Geometry check sheet. Reference: the model listing, model coordinates, mm. A direction names the side the tool comes from. Give positions to 0.01 mm unless a question says otherwise; leave off trailing zeros. Write each loop counter-clockwise with the first axis right and the second up, starting at its lowest first coordinate (ties: lowest second). Pieces come first, ordered by that corner, then holes. Notation, with made-up numbers: (52, 81.5) - (105, 81.5) arc R6 cw to (105, 87.5) - close; hole circle Ø2 at (-37.5, 50). An arc over 180 degrees is marked (long way). Use a Markdown table: item, result.
```python
from build123d import *

# Parameters (mm, degrees)
BOX_W             = 43
BOX_H             = 27
BOX_DEPTH         = 10
CYLINDER001_R     = 15.5
CYLINDER001_DEPTH = 9
CYLINDER002_R     = 17.5
CYLINDER002_DEPTH = 2
CYLINDER_R        = 3.5
CYLINDER_DEPTH    = 10
CYLINDER003_R     = 5.5
CYLINDER003_DEPTH = 2
CYLINDER004_R     = 5
CYLINDER004_DEPTH = 10
BOX001_W          = 35
BOX001_H          = 2
BOX001_DEPTH      = 2
CHAMFER_SIZE      = 1
CHAMFER001_SIZE   = 0.9
CHAMFER002_SIZE   = 1
CHAMFER003_SIZE   = 0.9
CHAMFER004_SIZE   = 0.5


with BuildPart() as cube:
    # Box → Box (new body)
    with BuildSketch(Plane(origin=(-22, 0, -1), x_dir=(1, 0, 0), z_dir=(0, 0, 1))):
        with Locations((21.5, 13.5)):
            Rectangle(BOX_W, BOX_H)
    extrude(amount=BOX_DEPTH)


with BuildPart() as cylinder001:
    # Cylinder001 → Cylinder001 (new body)
    with BuildSketch(Plane.XY.offset(-1)):
        Circle(CYLINDER001_R)
    extrude(amount=CYLINDER001_DEPTH)


with BuildPart() as cut001:
    # Cylinder002 → Cylinder002 (new body)
    with BuildSketch(Plane.XY):
        Circle(CYLINDER002_R)
    extrude(amount=CYLINDER002_DEPTH)

    # Cut: cut Cylinder001
    add(cylinder001.part, mode=Mode.SUBTRACT)

    # Cut001: cut Cube
    add(cube.part, mode=Mode.SUBTRACT)


with BuildPart() as cylinder:
    # Cylinder → Cylinder (new body)
    with BuildSketch(Plane.XY.offset(-3)):
        Circle(CYLINDER_R)
    extrude(amount=CYLINDER_DEPTH)


with BuildPart() as cut002:
    # Cylinder003 → Cylinder003 (new body)
    with BuildSketch(Plane.XY):
        Circle(CYLINDER003_R)
    extrude(amount=CYLINDER003_DEPTH)

    # Cut002: cut Cylinder
    add(cylinder.part, mode=Mode.SUBTRACT)


with BuildPart() as cylinder004:
    # Cylinder004 → Cylinder004 (new body)
    with BuildSketch(Plane.XY.offset(-3)):
        Circle(CYLINDER004_R)
    extrude(amount=CYLINDER004_DEPTH)


with BuildPart() as prop_guard:
    # Box001 → Box001 (new body)
    with BuildSketch(Plane(origin=(-17.5, -2, 0), x_dir=(1, 0, 0), z_dir=(0, 0, 1))):
        with Locations((17.5, 1)):
            Rectangle(BOX001_W, BOX001_H)
    extrude(amount=BOX001_DEPTH)

    # Cut003: cut Cylinder004
    add(cylinder004.part, mode=Mode.SUBTRACT)

    # Chamfer
    chamfer_edges = [prop_guard.edges().sort_by_distance(p)[0] for p in [
        (11.25, 0, 2),
    ]]
    chamfer(chamfer_edges, length=CHAMFER_SIZE)

    # Chamfer001
    chamfer001_edges = [prop_guard.edges().sort_by_distance(p)[0] for p in [
        (11.041288, -2, 2),
    ]]
    chamfer(chamfer001_edges, length=CHAMFER001_SIZE)

    # Chamfer002
    chamfer002_edges = [prop_guard.edges().sort_by_distance(p)[0] for p in [
        (-11.25, 0, 2),
    ]]
    chamfer(chamfer002_edges, length=CHAMFER002_SIZE)

    # Chamfer003
    chamfer003_edges = [prop_guard.edges().sort_by_distance(p)[0] for p in [
        (-11.041288, -2, 2),
    ]]
    chamfer(chamfer003_edges, length=CHAMFER003_SIZE)

    # Fusion: union Cut001, Cut002
    add(cut001.part)
    add(cut002.part)

    # Chamfer004
    chamfer004_edges = [prop_guard.edges().sort_by_distance(p)[0] for p in [
        (-3.5, 0, 0),
    ]]
    chamfer(chamfer004_edges, length=CHAMFER004_SIZE)


solid = prop_guard.part
```
1) Mould release check, pull along X, two halves, no side actions. Record for faces 1 (the cylindrical face through (17.498, -0.285, 1.715)), 2 (the flat face through (10.2, -1.6, 1.5)), 3 (the flat face through (0, -5, 2)): pulls with the +X half, pulls with the -X half, needs draft (parallel to the pull), parting line crosses it, or undercut.
Working result:
| item | result |
|---|---|
| face 1 | pulls with the +X half |
| face 2 | undercut |
| face 3 | needs draft |
2) Section check D-D on y = -13.5. Record the boundary of the cut face in (x, z), then the cut area to 3 significant figures.
Working result:
| item | result |
|---|---|
| outline | (-11.14, 0) - (-7.62, 0) - (-7.62, 2) - (-11.14, 2) - close; (7.62, 0) - (11.14, 0) - (11.14, 2) - (7.62, 2) - close |
| area | 14.1 mm² |
3) Section check B-B on y = -8.75. Record the boundary of the cut face in (x, z).
Working result:
| item | result |
|---|---|
| outline | (-15.16, 0) - (-12.79, 0) - (-12.79, 2) - (-15.16, 2) - close; (12.79, 0) - (15.16, 0) - (15.16, 2) - (12.79, 2) - close |
4) Section check C-C on x = -12. Record the boundary of the cut face in (y, z).
Working result:
| item | result |
|---|---|
| outline | (-12.74, 0) - (-9.81, 0) - (-9.81, 2) - (-12.74, 2) - close; (-2, 0) - (0, 0) - (0, 1) - (-1, 2) - (-1.1, 2) - (-2, 1.1) - close |
5) Set-up check for faces 4 (the flat face through (11.4, 0, 0.5)), 5 (the flat face through (-12.9, 0, 0.8)), 6 (the flat face through (-10.3, -2, 0.5)), 7 (the cylindrical face through (-15.498, -0.271, 1.715)): record each of +Z, -Z, +X, -X, +Y, -Y from which the full face is reachable in a straight line by a thin tool's end or side.
Working result:
| item | result |
|---|---|
| face 4 | +Z, -Z, +X, +Y |
| face 5 | +Z, -Z, -X, +Y |
| face 6 | +Z, -Z |
| face 7 | +Z, +Y |
6) Depth check by flat-ended pin: P1, Ø0.6, axis at x = 12.5, z = 1.5, coming from the +Y side; P2, Ø1, axis at x = -5.5, z = 0.5, coming from the +Y side; P3, Ø0.6, axis at x = -9, z = 0.5, coming from the -Y side. Enter the tip coordinate at first touch or a pass-through.
Working result:
| item | result |
|---|---|
| P1 | stops at y = -0.2 |
| P2 | stops at y = 2.29 |
| P3 | stops at y = -15.18 |
7) Section check A-A on x = 0. Record the boundary of the cut face in (y, z).
Working result:
| item | result |
|---|---|
| outline | (-17.5, 0) - (-15.5, 0) - (-15.5, 2) - (-17.5, 2) - close; (-5.5, 0) - (-4, 0) - (-3.5, 0.5) - (-3.5, 2) - (-5.5, 2) - close; (3.5, 0.5) - (4, 0) - (5.5, 0) - (5.5, 2) - (3.5, 2) - close |
8) Material ranges on L1, parallel to Y at x = 0, z = 1; L2, parallel to X at y = -0.5, z = 1.65; L3, parallel to Y at x = 3, z = 0.95, recorded low to high. Write a range as from..to.
Working result:
| item | result |
|---|---|
| L1 | y = -17.5..-15.5, -5.5..-3.5, 3.5..5.5 |
| L2 | x = -17.49..-15.49, -5.48..-3.46, 3.46..5.48, 15.49..17.49 |
| L3 | y = -17.24..-15.21, -4.61..-1.8, 1.8..4.61 |
